The listing builds one solid part. Answer for the finished solid, in the listing's coordinates (mm). A direction names the side the tool comes from. Round coordinates to 2 decimals unless told otherwise and drop trailing zeros. Write each loop counter-clockwise with the first axis right and the second up, starting at its lowest first coordinate (ties: lowest second). Pieces come first, ordered by that corner, then holes. Notation, with made-up numbers: (-33, 21) - (-24, 21) arc R11 cw to (-24, 35) - close; hole circle Ø4 at (22.5, 46.25). An arc over 180 degrees is marked (long way). Return JSON: item names as keys, results as strings. Group by question number.
(1) Section A-A, the plane x = 0 is taken. Write down the section's boundary in (y, z), then the cut area to 3 significant figures.
(2) Determine the mould class of faces 6 (the cylindrical face through (-8, 0, 17)), 7 (the cylindrical face through (8, 0, 17)), 8 (the cylindrical face through (-13.669, -0.526, 4.437)) for opening direction X: +X half, -X half, draft (parallel to the pull), parting line (faces both ways), or undercut.
(3) Each of these flat-tipped pins is pushed along its axis until it touches: pin 1 (5.5 mm diameter, centred on x = 12, y = 0, fed in from +Z); pin 2 (4 mm diameter, centred on y = -13, z = 16.5, fed in from +X); pin 3 (1.7 mm diameter, centred on y = 14, z = 17, fed in from -X). Where does it stop, or does it pass through?
(4) Which of the six approach directions +Z, -Z, +X, -X, +Y, -Y give full straight-line access (tool end or side, diameter ignored) to faces 1 (the flat face through (-14, 0, 9)), 2 (the flat face through (-4, 14, 17)), 3 (the flat face through (14, 4, 17)), 4 (the flat face through (4, -14, 17)), 5 (the flat face through (-7.4, -6.5, 15))?
(5) Section C-C, the plane z = 14.25 is taken. Write down the section's boundary in (x, y), then the cut area to 3 significant figures.
(6) Section B-B, the plane x = 11 is taken. Write down the section's boundary in (y, z).
(7) Find the intervals of material crossed by line 1 along Y through (x, z) = (0, 7.25); line 2 along Y through (x, z) = (10, 18.25); line 3 along Y through (x, z) = (12, 20.5), in increasing order. Write a range as [from, to].
(8) Section D-D, the plane z = 7.5 is taken. Write down the section's boundary in (x, y).
```python
from build123d import *

# Parameters (mm, degrees)
SKETCH1_R           = 16
SKETCH1_R_2         = 1.75
BOSS_EXTRUDE1_DEPTH = 24
SKETCH2_R           = 1.75
CUT_EXTRUDE1_DEPTH  = 33.984845005
SKETCH3_R           = 4
CUT_EXTRUDE2_DEPTH  = 15
CUT_EXTRUDE3_DEPTH  = 15


with BuildPart() as part:
    # Sketch1 → Boss-Extrude1 (new body)
    with BuildSketch(Plane.XY):
        Circle(SKETCH1_R)
        with Locations((0, 12)):
            Circle(SKETCH1_R_2, mode=Mode.SUBTRACT)
        with Locations((12, 0)):
            Circle(SKETCH1_R_2, mode=Mode.SUBTRACT)
        with Locations(Location((-12, 0, 0), (0, 0, 180))):
            Circle(SKETCH1_R_2, mode=Mode.SUBTRACT)
        with Locations(Location((0, -12, 0), (0, 0, 180))):
            Circle(SKETCH1_R_2, mode=Mode.SUBTRACT)
    extrude(amount=BOSS_EXTRUDE1_DEPTH)

    # Sketch2 → Cut-Extrude1 (cut, through all)
    with BuildSketch(Plane(origin=(0, 0, 0), x_dir=(-1, 0, 0), z_dir=(0, 0, -1))):
        with Locations((-5.656854249, 5.656854249)):
            Circle(SKETCH2_R)
        with Locations(Location((5.656854249, -5.656854249, 0), (0, 0, 180))):
            Circle(SKETCH2_R)
    extrude(amount=-CUT_EXTRUDE1_DEPTH, mode=Mode.SUBTRACT)

    # Sketch3 → Cut-Extrude2 (cut)
    with BuildSketch(Plane(origin=(0, 0, 0), x_dir=(-1, 0, 0), z_dir=(0, 0, -1))):
        with Locations((-5.656854249, 5.656854249)):
            Circle(SKETCH3_R)
        with Locations((5.656854249, -5.656854249)):
            Circle(SKETCH3_R)
    extrude(amount=-CUT_EXTRUDE2_DEPTH, mode=Mode.SUBTRACT)

    # Sketch4 → Cut-Extrude3 (cut)
    with BuildSketch(Plane.XY.offset(24)):
        with BuildLine():
            Line((-4, 12), (-4, 19.527532163))
            Line((-4, 19.527532163), (4, 19.527532163))
            Line((4, 19.527532163), (4, 12))
            ThreePointArc((4, 12), (0, 8), (-4, 12))
        make_face()
        with BuildLine():
            Line((12, 4), (20.319785819, 4))
            Line((20.319785819, 4), (20.319785819, -4))
            Line((20.319785819, -4), (12, -4))
            ThreePointArc((12, -4), (8, 0), (12, 4))
        make_face()
        with BuildLine():
            Line((-12, 4), (-20.860663916, 4))
            Line((-20.860663916, 4), (-20.860663916, -4))
            Line((-20.860663916, -4), (-12, -4))
            ThreePointArc((-12, -4), (-8, 0), (-12, 4))
        make_face()
        with BuildLine():
            Line((-4, -12), (-4, -17.609746143))
            Line((-4, -17.609746143), (4, -17.609746143))
            Line((4, -17.609746143), (4, -12))
            ThreePointArc((4, -12), (0, -8), (-4, -12))
        make_face()
    extrude(amount=-CUT_EXTRUDE3_DEPTH, mode=Mode.SUBTRACT)


solid = part.part
```
Working result:
{
 "1": {"outline": "(-16, 0) - (-13.75, 0) - (-13.75, 9) - (-16, 9) - close; (-10.25, 0) - (10.25, 0) - (10.25, 9) - (8, 9) - (8, 24) - (-8, 24) - (-8, 9) - (-10.25, 9) - close; (13.75, 0) - (16, 0) - (16, 9) - (13.75, 9) - close", "area": "465 mm^2"},
 "2": {"face 6": "-X half", "face 7": "+X half", "face 8": "undercut"},
 "3": {"pin 1": "stops at z = 9", "pin 2": "stops at x = 11.62", "pin 3": "stops at x = -9.11"},
 "4": {"face 1": "+Z, -X", "face 2": "+Z, +Y", "face 3": "+Z, +X", "face 4": "+Z, -Y", "face 5": "-Z"},
 "5": {"outline": "(-15.49, -4) arc R16 ccw to (-4, -15.49) - (-4, -12) arc R4 cw to (4, -12) - (4, -15.49) arc R16 ccw to (15.49, -4) - (12, -4) arc R4 cw to (12, 4) - (15.49, 4) arc R16 ccw to (4, 15.49) - (4, 12) arc R4 cw to (-4, 12) - (-4, 15.49) arc R16 ccw to (-15.49, 4) - (-12, 4) arc R4 cw to (-12, -4) - close; hole circle Ø8 at (-5.66, -5.66); hole circle Ø8 at (5.66, 5.66)", "area": "481 mm^2"},
 "6": {"outline": "(-11.62, 0) - (-1.44, 0) - (-1.44, 9) - (-3.87, 9) - (-3.87, 24) - (-11.62, 24) - close; (1.44, 0) - (11.62, 0) - (11.62, 24) - (3.87, 24) - (3.87, 9) - (1.44, 9) - close"},
 "7": {"line 1": "y = [-16, -13.75], [-10.25, 10.25], [13.75, 16]", "line 2": "y = [-12.49, -3.46], [3.46, 12.49]", "line 3": "y = [-10.58, -4], [4, 10.58]"},
 "8": {"outline": "circle Ø32 at (0, 0); hole circle Ø3.5 at (-12, 0); hole circle Ø8 at (-5.66, -5.66); hole circle Ø3.5 at (0, -12); hole circle Ø3.5 at (0, 12); hole circle Ø8 at (5.66, 5.66); hole circle Ø3.5 at (12, 0)"}
}
